The figure shows three views and two pictorial views of one solid part (mm, origin at its lowest corner). Answer the questions. A direction names the side the tool comes from. Round coordinates to 2 decimals unless told otherwise and drop trailing zeros. Order: outer loops, then holes, each group sorted by start corner. A loop starts at its lowest first (then second) coordinate and runs counter-clockwise, first axis right, second up. Notation, with made-up numbers: (11.5, 24) -> (59.5, 24) arc R19 ccw to (59.5, 37) -> close; hole circle Ø10 at (16.25, -19.5). An arc over 180 degrees is marked (long way). Return JSON: item names as keys, results as strings. Group by question number.
(1) Which of the six approach directions +Z, -Z, +X, -X, +Y, -Y give full straight-line access (tool end or side, diameter ignored) to the marked faces 1, 2 and 3?
(2) The part is cut by section A-A (x = 13.25). Determine the outline of the cut face in (y, z), plus the area to 3 significant figures.
(3) The part is cut by section B-B (z = 5.75). Determine the outline of the cut face in (x, y), plus the area to 3 significant figures.
(4) Consider line 1 (Y direction, x = 6.5, z = 7.75); line 2 (Y direction, x = 7.75, z = 7.5); line 3 (Z direction, x = 14.25, y = 105.5). Determine where each line is inside the solid, lowest interval first. Write a range as [from, to].
(5) Each of these flat-tipped pins is pushed along its axis until it touches: pin 1 (1.3 mm diameter, centred on y = 104, z = 6.5, fed in from -X); pin 2 (2 mm diameter, centred on y = 103, z = 6.5, fed in from +X); pin 3 (2 mm diameter, centred on y = 25.5, z = 4, fed in from +X). Where does it stop, or does it pass through?
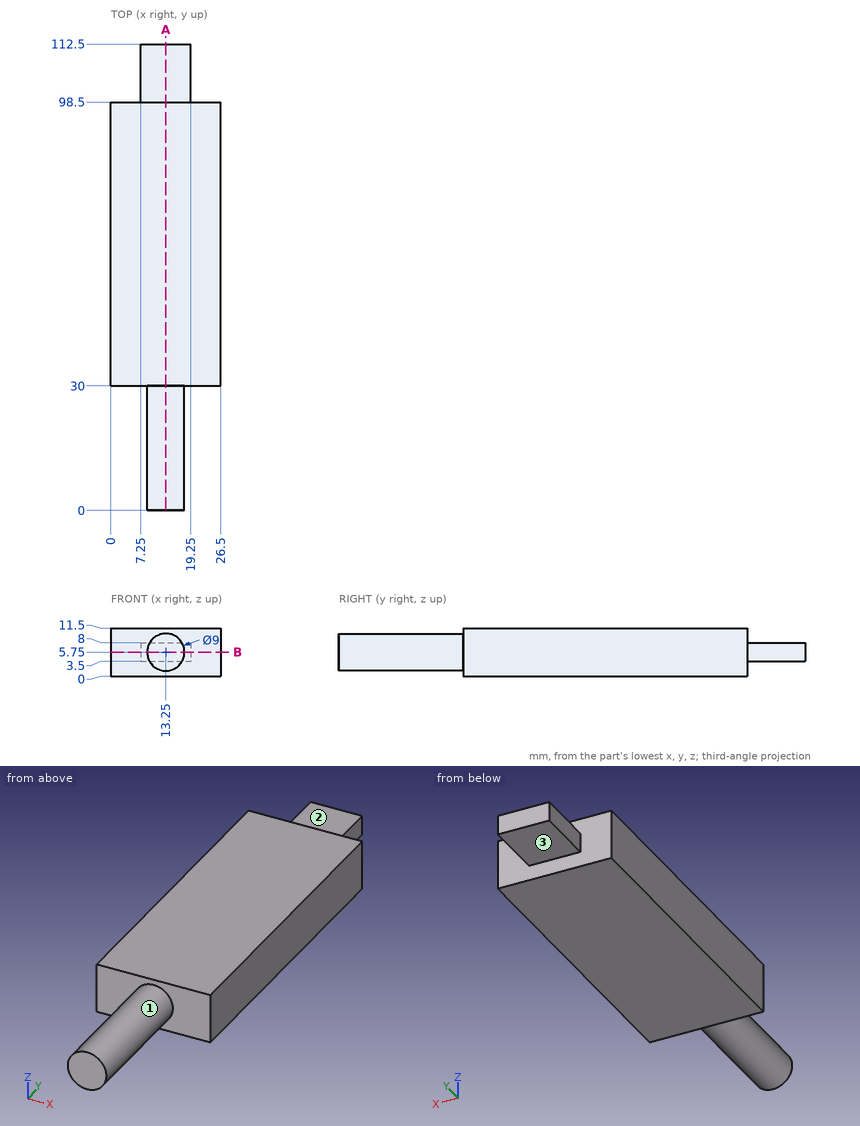
Answer below:
{
 "1": {"face 1": "-Y", "face 2": "+Z, +X, -X, +Y", "face 3": "-Z, +X, -X, +Y"},
 "2": {"outline": "(0, 1.25) -> (30, 1.25) -> (30, 0) -> (98.5, 0) -> (98.5, 3.5) -> (112.5, 3.5) -> (112.5, 8) -> (98.5, 8) -> (98.5, 11.5) -> (30, 11.5) -> (30, 10.25) -> (0, 10.25) -> close", "area": "1,120 mm²"},
 "3": {"outline": "(0, 30) -> (8.75, 30) -> (8.75, 0) -> (17.75, 0) -> (17.75, 30) -> (26.5, 30) -> (26.5, 98.5) -> (19.25, 98.5) -> (19.25, 112.5) -> (7.25, 112.5) -> (7.25, 98.5) -> (0, 98.5) -> close", "area": "2,250 mm²"},
 "4": {"line 1": "y = [30, 98.5]", "line 2": "y = [30, 112.5]", "line 3": "z = [3.5, 8]"},
 "5": {"pin 1": "stops at x = 7.25", "pin 2": "stops at x = 19.25", "pin 3": "stops at x = 17.69"}
}
